```python
from build123d import *

# Parameters (mm, degrees)
F0_R     = 1.27
F0_R_2   = 1.397
F0_R_3   = 3.556
F1_DEPTH = 3.175
F3_D     = 2.032
F5_D     = 4.318
F6_R     = 6.35


with BuildPart() as f1:
    # F0 (on Front) → F1 (new body)
    with BuildSketch(Plane.XZ):
        with BuildLine():
            Line((57.15, -12.7), (57.15, 12.7))
            Line((57.15, 12.7), (-57.15, 12.7))
            Line((-57.15, 12.7), (-57.15, -12.7))
            Line((-57.15, -12.7), (22.03733, -12.7))
            ThreePointArc((22.03733, -12.7), (35.247098, -14.447558), (47.548013, -19.569998))
            ThreePointArc((47.548013, -19.569998), (54.568108, -19.23657), (57.15, -12.7))
        make_face()
        with Locations((48.41875, -13.97)):
            Circle(F0_R, mode=Mode.SUBTRACT)
        with Locations((53.18125, -13.97)):
            Circle(F0_R, mode=Mode.SUBTRACT)
        with Locations((50.8, -9.2075)):
            Circle(F0_R, mode=Mode.SUBTRACT)
        with Locations((-50.8, 0)):
            Circle(F0_R_2, mode=Mode.SUBTRACT)
        Polygon((-25.908, 10.033), (14.986, 10.033), (14.986, -10.033), (-25.908, -10.033), (-25.908, -3.302), (-29.083, -3.302), (-29.083, 3.302), (-25.908, 3.302), align=None, mode=Mode.SUBTRACT)
        with Locations((50.8, 6.35)):
            Circle(F0_R_3, mode=Mode.SUBTRACT)
    extrude(amount=F1_DEPTH)

    # F3 (through all)
    with Locations(Plane.XZ.offset(3.175)):
        with Locations((-29.718, 5.08), (18.796, 5.08), (18.796, -5.08), (-29.718, -5.08)):
            Hole(F3_D / 2)

    # F5 (through all)
    with Locations(Plane(origin=(0, 0, 0), x_dir=(1, 0, 0), z_dir=(0, 1, 0))):
        with Locations((-36.703, 0), (26.797, 0)):
            Hole(F5_D / 2)

    # F6
    f6_edges = [f1.edges().sort_by_distance(p)[0] for p in [
        (-57.15, -1.5875, 12.7),
        (-57.15, -1.5875, -12.7),
        (57.15, -1.5875, 12.7),
        (57.15, -1.5875, -12.7),
    ]]
    fillet(f6_edges, radius=F6_R)


solid = f1.part
```
Geometry check sheet. Reference: the model listing, model coordinates, mm. A direction names the side the tool comes from. Give positions to 0.01 mm unless a question says otherwise; leave off trailing zeros. Order: outer loops, then holes, each group sorted by start corner. A loop starts at its lowest first (then second) coordinate and runs counter-clockwise, first axis right, second up. Notation, with made-up numbers: (81, 68.5) - (90, 68.5) arc R20 ccw to (90, 96.5) - close; hole circle Ø2 at (-23.5, -36). An arc over 180 degrees is marked (long way). Write item = value, one per line. Start each with the question number.
1) Section check D-D (y = -0.65). Count the separate pieces of the cut face and the enclosed holes in it, then the cut area to 3 significant figures.
2) Section check A-A (z = 0). Enter the section's corners in (x, y) (3 decimals), then the cut area to 3 significant figures.
3) Section check C-C (z = -5.08). Enter the section's corners in (x, y) (3 decimals), then the cut area to 3 significant figures.
4) Section check B-B (x = -6.5). Enter the section's corners in (y, z) (3 decimals), then the cut area to 3 significant figures.
5) Draft check along X on faces 3 (the cylindrical face through (-55.34, -1.61, -10.79)), 4 (the flat face through (-25.908, -2, -7)), 5 (the flat face through (-15, -2, -12.7)). Enter one of: released by +X, released by -X, zero draft, split by the parting line, or undercut.
6) Access from +Z, -Z, +X, -X, +Y, -Y to the whole of each face (thin tool, end or side, straight path). Record for faces 1 (the cylindrical face through (55.34, -1.61, 10.79)), 2 (the flat face through (-5, -2, -10.033)).
7) Scan lines: L1, parallel to Z at x = -17, y = -2.1; L2, parallel to X at y = -1.1, z = -3.5; L3, parallel to X at y = -1.65, z = -9.5. Record each from-to range of solid material in increasing order.
8) Gauge pin test, flat ends, axial feed: pin 1 Ø2.5 at (x, z) = (-50.8, 0) entering from +Y; pin 2 Ø1.5 at (y, z) = (-2.5, 3) entering from +X; pin 3 Ø1.6 at (x, y) = (-26.5, -1.5) entering from -Z. Record the tip position at first contact, or that the pin passes through.
Geometry check:
q1.separate_pieces = 1
q1.enclosed_holes = 12
q1.area = 2,050 mm2
q2.outline = (-57.15, -3.175) - (-52.197, -3.175) - (-52.197, 0) - (-57.15, 0) - close; (-49.403, -3.175) - (-38.862, -3.175) - (-38.862, 0) - (-49.403, 0) - close; (-34.544, -3.175) - (-29.083, -3.175) - (-29.083, 0) - (-34.544, 0) - close; (14.986, -3.175) - (24.638, -3.175) - (24.638, 0) - (14.986, 0) - close; (28.956, -3.175) - (57.15, -3.175) - (57.15, 0) - (28.956, 0) - close
q2.area = 187 mm2
q3.outline = (-57.15, -3.175) - (-30.734, -3.175) - (-30.734, 0) - (-57.15, 0) - close; (-28.702, -3.175) - (-25.908, -3.175) - (-25.908, 0) - (-28.702, 0) - close; (14.986, -3.175) - (17.78, -3.175) - (17.78, 0) - (14.986, 0) - close; (19.812, -3.175) - (57.15, -3.175) - (57.15, 0) - (19.812, 0) - close
q3.area = 220 mm2
q4.outline = (-3.175, -12.7) - (0, -12.7) - (0, -10.033) - (-3.175, -10.033) - close; (-3.175, 10.033) - (0, 10.033) - (0, 12.7) - (-3.175, 12.7) - close
q4.area = 16.9 mm2
q5.face_3 = released by -X
q5.face_4 = undercut
q5.face_5 = zero draft
q6.face_1 = +Z, +X, +Y, -Y
q6.face_2 = +Y, -Y
q7.L1 = -12.7 to -10.03, 10.03 to 12.7
q7.L2 = -57.15 to -25.91, 14.99 to 57.15
q7.L3 = -56.31 to -25.91, 14.99 to 49.56, 52.04 to 57.15
q8.pin_1 = through
q8.pin_2 = 57.15
q8.pin_3 = -12.7
